from build123d import *

# Parameters (mm, degrees)
BOSS_EXTRUDE1_START = 2
SKETCH2_W           = 28
SKETCH2_H           = 14
SKETCH2_R           = 2.85
BOSS_EXTRUDE1_DEPTH = 8.1
BOSS_EXTRUDE5_DEPTH = 28
CUT_EXTRUDE1_REACH  = 83.112
SKETCH7_R           = 1.475
SKETCH7_W           = 15.52
SKETCH7_H           = 20.32
BOSS_EXTRUDE7_DEPTH = 2
FILLET1_R           = 2
BOSS_EXTRUDE8_START = -2
BOSS_EXTRUDE8_DEPTH = 6.386
FILLET2_R           = 0.5


with BuildPart() as part:
    # Sketch2 → Boss-Extrude1 (new body)
    with BuildSketch(Plane.XY.offset(BOSS_EXTRUDE1_START)):
        with Locations((-62.5, -8)):
            Rectangle(SKETCH2_W, SKETCH2_H)
        with Locations((-54.5, -8.9)):
            Circle(SKETCH2_R, mode=Mode.SUBTRACT)
        with Locations((-70.5, -8.9)):
            Circle(SKETCH2_R, mode=Mode.SUBTRACT)
    extrude(amount=BOSS_EXTRUDE1_DEPTH)

    # Sketch6 → Boss-Extrude5 (add)
    with BuildSketch(Plane.ZY.offset(76.5)):
        Polygon((10.1, -15), (14.656017135, -15), (19.003880422, -13.331011655), (22.5, 13.224653006), (19.240190464, 17.015911609), (17.723687023, 15.711987794), (19.525665416, 13.616231583), (16.26251061, -11.169889951), (14.1, -12), (10.1, -12), align=None)
    extrude(amount=-BOSS_EXTRUDE5_DEPTH)

    # Sketch7 → Cut-Extrude1 (cut, up to next)
    with BuildSketch(Plane(origin=(0, -2.686404695, 20.405269514), x_dir=(1, 0, 0), z_dir=(0, -0.13052619222004436, 0.9914448613738114)), mode=Mode.PRIVATE) as cut_extrude1_sk1:
        with Locations(Location((-54.716, -4.710052631, 0), (0, 0, 270))):
            Circle(SKETCH7_R)
    cut_extrude1_tool1 = extrude(cut_extrude1_sk1.sketch, amount=-CUT_EXTRUDE1_REACH, mode=Mode.PRIVATE) & part.part
    # Sketch7 → Cut-Extrude1 (cut, up to next)
    with BuildSketch(Plane(origin=(0, -2.686404695, 20.405269514), x_dir=(1, 0, 0), z_dir=(0, -0.13052619222004436, 0.9914448613738114)), mode=Mode.PRIVATE) as cut_extrude1_sk2:
        with Locations(Location((-54.716, 10.529947369, 0), (0, 0, 270))):
            Circle(SKETCH7_R)
    cut_extrude1_tool2 = extrude(cut_extrude1_sk2.sketch, amount=-CUT_EXTRUDE1_REACH, mode=Mode.PRIVATE) & part.part
    # Sketch7 → Cut-Extrude1 (cut, up to next)
    with BuildSketch(Plane(origin=(0, -2.686404695, 20.405269514), x_dir=(1, 0, 0), z_dir=(0, -0.13052619222004436, 0.9914448613738114)), mode=Mode.PRIVATE) as cut_extrude1_sk3:
        with Locations((-64.646, 2.909947369)):
            Rectangle(SKETCH7_W, SKETCH7_H)
    cut_extrude1_tool3 = extrude(cut_extrude1_sk3.sketch, amount=-CUT_EXTRUDE1_REACH, mode=Mode.PRIVATE) & part.part
    add(cut_extrude1_tool1.solids().sort_by_distance((-54.716, -7.356162, 19.790484))[0], mode=Mode.SUBTRACT)
    add(cut_extrude1_tool2.solids().sort_by_distance((-54.716, 7.753458, 21.779703))[0], mode=Mode.SUBTRACT)
    add(cut_extrude1_tool3.solids().sort_by_distance((-64.646, 0.198648, 20.785094))[0], mode=Mode.SUBTRACT)

    # Sketch10 → Boss-Extrude7 (add)
    with BuildSketch(Plane(origin=(-48.5, 0, 0), x_dir=(0, 0, -1), z_dir=(1, 0, 0))):
        Polygon((-18.13225899, 3.03225899), (-17.67742093, -0.42257907), (-10.1, -8), (-10.1, -5), align=None)
    extrude(amount=-BOSS_EXTRUDE7_DEPTH)

    # Fillet1
    # the kernel refuses this fillet: 2 mm, written as the material it takes off along each edge
    with BuildSketch(Plane(origin=(-50.5, 12.598930148, 20.400364102), x_dir=(0, 0.6519619071782031, 0.758251720465282), z_dir=(1, 0, 0))) as fillet1_piece_1_section:
        Polygon((0, 0), (FILLET1_R * 1.02, 0), (FILLET1_R * 1.02, FILLET1_R * 0.45615786741), (FILLET1_R * 0.68, FILLET1_R * 0.76026311235), align=None)
    fillet1_piece_1 = extrude(amount=FILLET1_R * 1.02, mode=Mode.PRIVATE)
    fillet1_piece_1 = fillet1_piece_1 - Plane(origin=(-50.5, 12.598930148, 20.400364102), x_dir=(0, -0.28560210337141756, -0.9583482866629555), z_dir=(1, 0, 0)) * Sphere(FILLET1_R, mode=Mode.PRIVATE)
    add(fillet1_piece_1, mode=Mode.SUBTRACT)
    with BuildSketch(Plane(origin=(-74.5, 12.598930148, 20.400364102), x_dir=(0, 0.6519619071782031, 0.758251720465282), z_dir=(-1, 0, 0))) as fillet1_piece_2_section:
        Polygon((0, 0), (FILLET1_R * 1.02, 0), (FILLET1_R * 1.02, -FILLET1_R * 0.45615786741), (FILLET1_R * 0.68, -FILLET1_R * 0.76026311235), align=None)
    fillet1_piece_2 = extrude(amount=FILLET1_R * 1.02, mode=Mode.PRIVATE)
    fillet1_piece_2 = fillet1_piece_2 - Plane(origin=(-74.5, 12.598930148, 20.400364102), x_dir=(0, -0.28560210337141756, -0.9583482866629555), z_dir=(-1, 0, 0)) * Sphere(FILLET1_R, mode=Mode.PRIVATE)
    add(fillet1_piece_2, mode=Mode.SUBTRACT)
    with BuildSketch(Plane(origin=(-76.5, -15, 19.656017135), x_dir=(1, 0, 0), z_dir=(0, 0, -1)), Plane(origin=(-48.5, -15, -3), x_dir=(-1, 0, 0), z_dir=(0, 0, 1))) as fillet1_piece_3:
        with BuildLine():
            CenterArc((FILLET1_R, -FILLET1_R), FILLET1_R, 90, 90)
            Line((0, -FILLET1_R), (0, 0))
            Line((0, 0), (FILLET1_R, 0))
        make_face()
    extrude(amount=22.656017135, mode=Mode.SUBTRACT)
    with BuildSketch(Plane(origin=(-76.5, -1, -3), x_dir=(0, -1, 0), z_dir=(0, 0, 1))) as fillet1_piece_4:
        with BuildLine():
            CenterArc((FILLET1_R, FILLET1_R), FILLET1_R, 180, 90)
            Line((0, FILLET1_R), (0, 0))
            Line((0, 0), (FILLET1_R, 0))
        make_face()
    extrude(amount=18.1, mode=Mode.SUBTRACT)
    with BuildSketch(Plane(origin=(-48.5, -1, -3), x_dir=(0, -1, 0), z_dir=(0, 0, 1))) as fillet1_piece_5_section:
        with BuildLine():
            CenterArc((FILLET1_R, -FILLET1_R), FILLET1_R, 90, 90)
            Line((0, -FILLET1_R), (0, 0))
            Line((0, 0), (FILLET1_R, 0))
        make_face()
    fillet1_piece_5 = extrude(amount=18.1, mode=Mode.PRIVATE)
    fillet1_piece_5 = split(fillet1_piece_5, bisect_by=Plane(origin=(-48.946735878, -5.248367939, 9.851632061), z_dir=(0, 0.707106781186545, -0.7071067811865501)), keep=Keep.TOP, mode=Mode.PRIVATE)
    add(fillet1_piece_5, mode=Mode.SUBTRACT)
    with BuildSketch(Plane(origin=(-48.5, 13.902853963, 21.916867543), x_dir=(0, -0.6519619071782031, -0.758251720465282), z_dir=(0, 0.758251720465282, -0.6519619071782031))) as fillet1_piece_6:
        with BuildLine():
            CenterArc((FILLET1_R, FILLET1_R), FILLET1_R, 180, 90)
            Line((0, FILLET1_R), (0, 0))
            Line((0, 0), (FILLET1_R, 0))
        make_face()
    extrude(amount=9.105572809, mode=Mode.SUBTRACT)
    with BuildSketch(Plane(origin=(-76.5, 13.902853963, 21.916867543), x_dir=(0, -0.6519619071782031, -0.758251720465282), z_dir=(0, 0.758251720465282, -0.6519619071782031))) as fillet1_piece_7:
        with BuildLine():
            CenterArc((FILLET1_R, -FILLET1_R), FILLET1_R, 90, 90)
            Line((0, -FILLET1_R), (0, 0))
            Line((0, 0), (FILLET1_R, 0))
        make_face()
    extrude(amount=9.105572809, mode=Mode.SUBTRACT)
    with BuildSketch(Plane(origin=(-48.5, -18.288235962, 18.351249461), x_dir=(0, 0.1305261922200442, -0.9914448613738114), z_dir=(0, 0.9914448613738114, 0.13052619222004422))) as fillet1_piece_8:
        with BuildLine():
            CenterArc((FILLET1_R, FILLET1_R), FILLET1_R, 180, 90)
            Line((0, FILLET1_R), (0, 0))
            Line((0, 0), (FILLET1_R, 0))
        make_face()
    extrude(amount=30.890385254, mode=Mode.SUBTRACT)
    with BuildSketch(Plane(origin=(-76.5, -18.288235962, 18.351249461), x_dir=(0, 0.1305261922200442, -0.9914448613738114), z_dir=(0, 0.9914448613738114, 0.13052619222004422))) as fillet1_piece_9:
        with BuildLine():
            CenterArc((FILLET1_R, -FILLET1_R), FILLET1_R, 90, 90)
            Line((0, -FILLET1_R), (0, 0))
            Line((0, 0), (FILLET1_R, 0))
        make_face()
    extrude(amount=30.890385254, mode=Mode.SUBTRACT)
    with BuildSketch(Plane(origin=(-74.5, 13.224653006, 22.5), x_dir=(0, 0.7582517204652818, -0.6519619071782033), z_dir=(1, 0, 0))) as fillet1_piece_10:
        with BuildLine():
            CenterArc((FILLET1_R * 0.4472135955, -FILLET1_R), FILLET1_R, 90, 48.189685104)
            Line((-FILLET1_R * 0.298142397, -FILLET1_R * 0.333333333333), (0, 0))
            Line((0, 0), (FILLET1_R * 0.4472135955, 0))
        make_face()
    extrude(amount=24, mode=Mode.SUBTRACT)
    with BuildSketch(Plane(origin=(-48.5, 20.275721145, 23.031449066), x_dir=(0, -0.7582517204652808, 0.6519619071782047), z_dir=(0, -0.6519619071782047, -0.7582517204652808))) as fillet1_piece_11:
        with BuildLine():
            CenterArc((FILLET1_R, FILLET1_R), FILLET1_R, 180, 90)
            Line((0, FILLET1_R), (0, 0))
            Line((0, 0), (FILLET1_R, 0))
        make_face()
    extrude(amount=12, mode=Mode.SUBTRACT)
    with BuildSketch(Plane(origin=(-76.5, 20.275721145, 23.031449066), x_dir=(0, -0.7582517204652808, 0.6519619071782046), z_dir=(0, -0.6519619071782047, -0.7582517204652808))) as fillet1_piece_12:
        with BuildLine():
            CenterArc((FILLET1_R, -FILLET1_R), FILLET1_R, 90, 90)
            Line((0, -FILLET1_R), (0, 0))
            Line((0, 0), (FILLET1_R, 0))
        make_face()
    extrude(amount=12, mode=Mode.SUBTRACT)

    # Sketch11 → Boss-Extrude8 (add)
    with BuildSketch(Plane(origin=(-48.5, 0, 0), x_dir=(0, 0, -1), z_dir=(1, 0, 0)).offset(BOSS_EXTRUDE8_START)):
        Polygon((-21.159704036, 3.044094423), (-23.468909239, 5.261654192), (-21.486019516, 5.522706576), align=None)
        Polygon((-22.399702862, 12.462820606), (-22.073387381, 9.984208452), (-24.056277104, 9.723156068), align=None)
        Polygon((-21.479690069, -9.847965496), (-19.496800347, -9.586913111), (-19.170484866, -12.065525265), align=None)
        Polygon((-22.067057934, -5.386463619), (-20.084168212, -5.125411235), (-20.410483692, -2.646799082), align=None)
    extrude(amount=-BOSS_EXTRUDE8_DEPTH)

    # Fillet2
    fillet2_edges = [part.edges().sort_by_distance(p)[0] for p in [
        (-53.693, 5.261654192, 23.468909239),
        (-53.693, 9.723156068, 24.056277104),
        (-53.693, -5.386463619, 22.067057934),
        (-53.693, -9.847965496, 21.479690069),
    ]]
    fillet(fillet2_edges, radius=FILLET2_R)


solid = part.part
Work out the finished part from the listing and answer in its coordinate system (mm). A direction names the side the tool comes from. Give positions to 0.01 mm unless a question says otherwise; leave off trailing zeros. Order: outer loops, then holes, each group sorted by start corner. A loop starts at its lowest first (then second) coordinate and runs counter-clockwise, first axis right, second up. Notation, with made-up numbers: (6.25, 56.25) -> (21.25, 56.25) arc R15 ccw to (21.25, 81.25) -> close; hole circle Ø9 at (-8, 89). An arc over 180 degrees is marked (long way). Answer as a JSON object with one key per item and string values. Group by question number.
1. Section D-D on x = -55.5 is taken. Count the separate pieces of the cut face and the enclosed holes in it, plus the area to 3 significant figures.
2. Section C-C on x = -70.5 is taken. Determine the outline of the cut face in (y, z), plus the area to 3 significant figures.
3. Section A-A on x = -62.5 is taken. Determine the outline of the cut face in (y, z), plus the area to 3 significant figures.
4. Flat-ended cylindrical pins translate along their axes: pin 1 Ø1.5 at (x, z) = (-63, 6) entering from +Y; pin 2 Ø1 at (x, z) = (-71.5, 12.5) entering from +Y; pin 3 Ø8 at (x, z) = (-54, 19.5) entering from -Y; pin 4 Ø4.5 at (y, z) = (0, 20.5) entering from +X. Find the tip coordinate at first contact, or state that the pin passes through.
5. Consider line 1 along Y through (x, z) = (-54.5, 8); line 2 along Z through (x, y) = (-60.25, -4); line 3 along Y through (x, z) = (-73.5, 6.25). Determine where each line is inside the solid, lowest interval first. Write a range as [from, to].
6. A tool of negligible diameter and unlimited length cuts with its end or side. For faces 5 (the flat face through (-53.648, 3.782, 21.928)), 6 (the flat face through (-50.5, 11, 23)), 7 (the cylindrical face through (-49.07, -1.6, 5.99)), 8 (the flat face through (-53.648, 9.922, 22.542)), from which of +Z, -Z, +X, -X, +Y, -Y can it reach the whole face along a straight path? Write none if from no direction.
7. The mould has two halves that part along X. Classify faces 1 (the cylindrical face through (-75.9, -14.43, 9.98)), 2 (the cylindrical face through (-51.782, -8.044, 5.993)), 3 (the flat face through (-63, -1, 6)), 4 (the cylindrical face through (-56.156, -6.846, 18.366)): released by +X, released by -X, zero draft, split by the parting line, or undercut.
8. Section B-B on z = 12 is taken. Determine the outline of the cut face in (x, y).
Result sheet:
{
 "1": {"separate pieces": "4", "enclosed holes": "0", "area": "173 mm^2"},
 "2": {"outline": "(-15, 2) -> (-11.75, 2) -> (-11.75, 10.1) -> (-12, 10.1) -> (-12, 14.1) -> (-11.17, 16.26) -> (-9.48, 16.48) -> (-9.87, 19.46) -> (-13.33, 19) -> (-15, 14.66) -> close; (-6.05, 2) -> (-1, 2) -> (-1, 10.1) -> (-6.05, 10.1) -> close; (10.27, 22.11) -> (10.66, 19.14) -> (13.62, 19.53) -> (15.71, 17.72) -> (17.02, 19.24) -> (13.9, 21.92) arc R2 ccw to (12.34, 22.38) -> close", "area": "115 mm^2"},
 "3": {"outline": "(-15, 2) -> (-1, 2) -> (-1, 10.1) -> (-12, 10.1) -> (-12, 14.1) -> (-11.17, 16.26) -> (-9.48, 16.48) -> (-9.87, 19.46) -> (-13.33, 19) -> (-15, 14.66) -> close; (10.27, 22.11) -> (10.66, 19.14) -> (13.62, 19.53) -> (15.71, 17.72) -> (17.02, 19.24) -> (13.9, 21.92) arc R2 ccw to (12.34, 22.38) -> close", "area": "161 mm^2"},
 "4": {"pin 1": "stops at y = -1", "pin 2": "stops at y = -12", "pin 3": "stops at y = -14.68", "pin 4": "stops at x = -48.5"},
 "5": {"line 1": "y = [-15, -11.75], [-6.05, -1]", "line 2": "z = [2, 10.1]", "line 3": "y = [-15, -1]"},
 "6": {"face 5": "+Z, +X, -X", "face 6": "+Z, +X, -Y", "face 7": "-Z, +X, +Y", "face 8": "+X, -X"},
 "7": {"face 1": "released by -X", "face 2": "undercut", "face 3": "zero draft", "face 4": "undercut"},
 "8": {"outline": "(-76.5, -13) arc R2 ccw to (-74.5, -15) -> (-50.5, -15) arc R2 ccw to (-48.5, -13) -> (-48.5, -12) -> (-76.5, -12) -> close; (-50.5, -6.1) -> (-48.5, -6.1) -> (-48.5, -3.1) -> (-50.5, -3.1) -> close"}
}
